Can you work these out from the drawing? Everything is in mm from the part's minimum corner. Coordinates: 2 decimals unless noted, no trailing zeros. Write each loop counter-clockwise with the first axis right and the second up, starting at its lowest first coordinate (ties: lowest second). Pieces come first, ordered by that corner, then holes. Notation, with made-up numbers: M 86.25,46.25 L 127.25,46.25 A28 cw 127.25,79.25 Z; hole C 20.25,16.25 d1. An arc over 180 degrees is marked long. Write item = value, one per line.
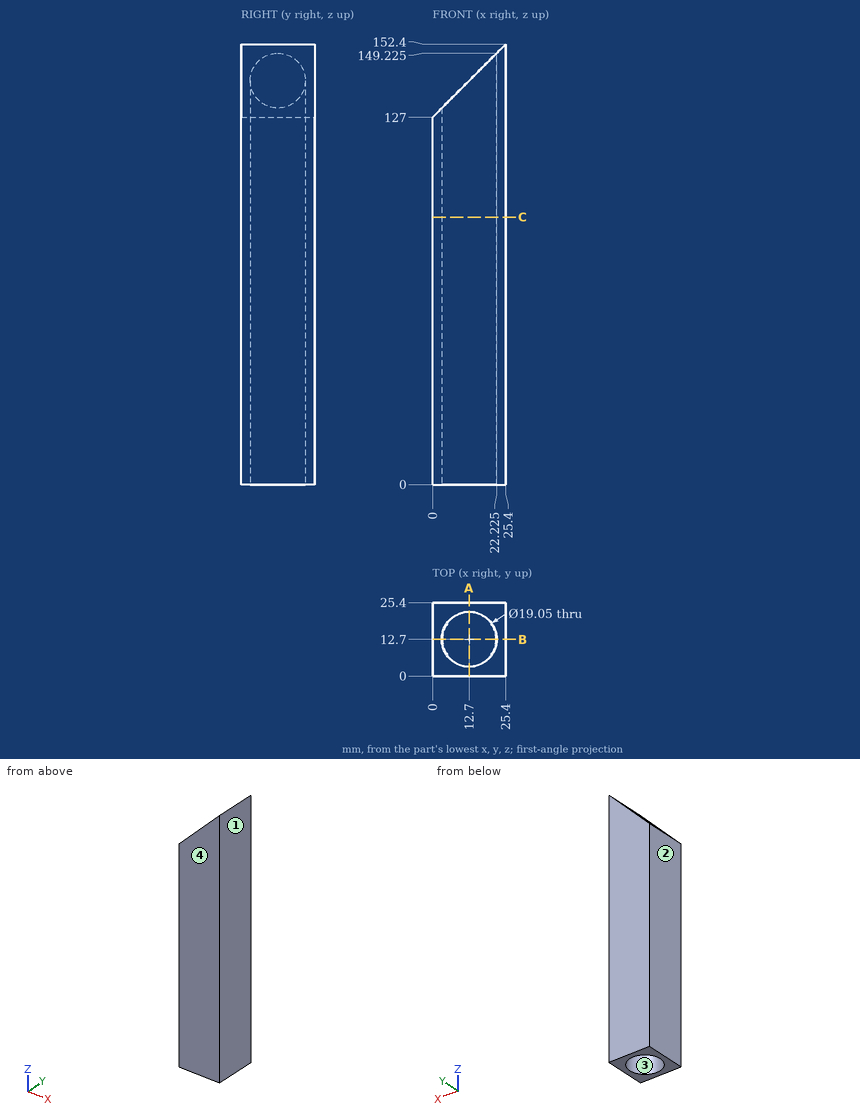
Item 1: Imagine slicing it at C-C (z = 92.5). Write out the boundary of the cut face in (x, y) (3 decimals).
Numbers:
outline = M 0,0 L 25.4,0 L 25.4,25.4 L 0,25.4 Z; hole C 12.7,12.7 d19.05
Item 2: If we mould it in two halves opening along X, with no side actions, what happens to the marked faces 1, 2, 3 and 4? For each: pulls with the +X half, pulls with the -X half, needs draft (parallel to the pull), parting line crosses it, or undercut.
Numbers:
face_1 = pulls with the +X half
face_2 = pulls with the -X half
face_3 = undercut
face_4 = needs draft
Item 3: If I drill on line 1 along X through (y, z) = (12.7, 52) (3 decimals); line 2 along Y through (x, z) = (5, 77.5), over which ranges is the centre line in solid material (lowest first)?
Numbers:
line_1 = 0 to 3.175, 22.225 to 25.4
line_2 = 0 to 7.09, 18.31 to 25.4
Item 4: Imagine slicing it at A-A (x = 12.7). Write out the boundary of the cut face in (y, z) (3 decimals).
Numbers:
outline = M 0,0 L 3.175,0 L 3.175,139.7 L 0,139.7 Z; M 22.225,0 L 25.4,0 L 25.4,139.7 L 22.225,139.7 Z
Item 5: Imagine slicing it at B-B (y = 12.7). Write out the boundary of the cut face in (x, z) (3 decimals), and give its area (3 significant figures).
Numbers:
outline = M 0,0 L 3.175,0 L 3.175,130.175 L 0,127 Z; M 22.225,0 L 25.4,0 L 25.4,152.4 L 22.225,149.225 Z
area = 887 mm²
